from build123d import *

# Parameters (mm, degrees)
SKETCH1_W                = 15.621
SKETCH1_H                = 20.193
SKETCH1_R                = 1.7145
BOSS_EXTRUDE1_DEPTH      = 1.3
SKETCH2_R                = 1.7145
BOSS_EXTRUDE2_DEPTH      = 3.6
BOSS_EXTRUDE2_DRAFT      = 3
SKETCH3_W                = 2
SKETCH3_H                = 2.155291512
SKETCH3_H_2              = 4
SKETCH3_W_2              = 1.5
SKETCH3_H_3              = 2.998822354
BOSS_EXTRUDE3_DEPTH      = 0.3
BOSS_EXTRUDE3_DEPTH_BACK = 0.3


with BuildPart() as part:
    # Sketch1 → Boss-Extrude1 (new body)
    with BuildSketch(Plane(origin=(0, 0, 0), x_dir=(1, 0, 0), z_dir=(0, 1, 0))):
        with Locations((7.8105, 10.0965)):
            Rectangle(SKETCH1_W, SKETCH1_H)
        with Locations((7.8105, 14.4785)):
            Circle(SKETCH1_R, mode=Mode.SUBTRACT)
    extrude(amount=BOSS_EXTRUDE1_DEPTH)


with BuildPart() as boss_extrude2_tool:
    # Sketch2 → Boss-Extrude2 (with draft: the straight prism first)
    with BuildSketch(Plane(origin=(0, 1.3, 0), x_dir=(1, 0, 0), z_dir=(0, 1, 0))):
        with BuildLine():
            Line((15.621, 20.193), (0, 20.193))
            Line((0, 20.193), (0, 17.3995))
            ThreePointArc((0, 17.3995), (2.065458908, 16.543958908), (2.921, 14.4785))
            ThreePointArc((2.921, 14.4785), (2.065458908, 12.413041092), (0, 11.5575))
            Line((0, 11.5575), (0, 0))
            Line((0, 0), (15.621, 0))
            Line((15.621, 0), (15.621, 11.5575))
            ThreePointArc((15.621, 11.5575), (12.7, 14.4785), (15.621, 17.3995))
            Line((15.621, 17.3995), (15.621, 20.193))
        make_face()
        with Locations((7.8105, 14.4785)):
            Circle(SKETCH2_R, mode=Mode.SUBTRACT)
    extrude(amount=BOSS_EXTRUDE2_DEPTH)
    # Boss-Extrude2: the draft: its side faces are tilted about the plane it starts from
    boss_extrude2_sides = [boss_extrude2_tool.faces().sort_by_distance(p)[0] for p in [
        (15.621, 3.1, -18.79625),
        (6.096, 3.1, -14.4785),
        (15.621, 3.1, -5.77875),
        (7.8105, 3.1, 0),
        (0, 3.1, -5.77875),
        (2.921, 3.1, -14.4785),
        (0, 3.1, -18.79625),
        (7.8105, 3.1, -20.193),
        (12.7, 3.1, -14.4785),
    ]]
    draft(boss_extrude2_sides, Plane(origin=(0, 1.3, 0), x_dir=(1, 0, 0), z_dir=(0, 1, 0)), BOSS_EXTRUDE2_DRAFT)


with BuildPart() as part_1:
    add(part.part)

    # Boss-Extrude2: add boss_extrude2_tool
    add(boss_extrude2_tool.part)

    # Sketch3 → Boss-Extrude3 (add, two sides)
    with BuildSketch(Plane(origin=(0, 2.45, 0), x_dir=(1, 0, 0), z_dir=(0, 1, 0))) as boss_extrude3_sk:
        with Locations((2.8105, 1.077645756)):
            Rectangle(SKETCH3_W, SKETCH3_H)
        with Locations((2.8105, -2)):
            Rectangle(SKETCH3_W, SKETCH3_H_2)
        with Locations((12.8105, 1.077645756)):
            Rectangle(SKETCH3_W, SKETCH3_H)
        with Locations((12.8105, -2)):
            Rectangle(SKETCH3_W, SKETCH3_H_2)
        with Locations((7.0605, 1.499411177)):
            Rectangle(SKETCH3_W_2, SKETCH3_H_3)
        Polygon((7.8105, 0), (6.3105, 0), (6.3105, -4), (9.3105, -4), (9.3105, 0), align=None)
        with Locations((8.5605, 1.499411177)):
            Rectangle(SKETCH3_W_2, SKETCH3_H_3)
    extrude(amount=BOSS_EXTRUDE3_DEPTH)
    extrude(boss_extrude3_sk.sketch, amount=-BOSS_EXTRUDE3_DEPTH_BACK)


solid = part_1.part
Can you work these out from the model? Positions are in its coordinate system, mm. A direction names the side the tool comes from. Coordinates: 2 decimals unless noted, no trailing zeros. Order: outer loops, then holes, each group sorted by start corner. A loop starts at its lowest first (then second) coordinate and runs counter-clockwise, first axis right, second up. Notation, with made-up numbers: M -39,1.5 L -11,1.5 A25 ccw -11,16.5 Z; hole C 36,11 d8. An arc over 180 degrees is marked long. Write item = value, one per line.
(1) Suppose I cut it at C-C on y = 0.8. Please give me the cut outline in (x, z) (1 decimal).
Results are:
outline = M 0,-20.2 L 15.6,-20.2 L 15.6,0 L 0,0 Z; hole C 7.8,-14.5 d3.4
(2) I need wall thicknesses on line 1 along X through (y, z) = (2.55, -15.5); line 2 along Z through (x, y) = (14, 2.35); line 3 along Z through (x, y) = (13.25, 2.8). Which ranges of each line are inside material? Lowest first, please. Write a range as [from, to].
Results are:
line_1 = [2.81, 6.35], [9.27, 12.81]
line_2 = [-20.14, -16.97], [-11.98, -0.06]
line_3 = [-20.11, -16.32], [-12.64, -0.08]
(3) If we mould it in two halves opening along Z, with no side actions, what happens to faces 5 (the face through (8.602, 0.641, -12.957)), 6 (the face through (13, 2.75, 2)), 7 (the face through (8, 1, -20.193)), 8 (the face through (12.61, 3.07, -14.41))? For each: pulls with the +Z half, pulls with the -Z half, needs draft (parallel to the pull), parting line crosses it, or undercut.
Results are:
face_5 = undercut
face_6 = needs draft
face_7 = pulls with the -Z half
face_8 = undercut
(4) For faces 1 (the face through (1, 1.3, -15)), 2 (the face through (3, 2.75, 2)), 3 (the face through (15.53, 3.07, -5.7)), 4 (the face through (8, 1, 0)), which set-ups out of +Z, -Z, +X, -X, +Y, -Y let a thin tool reach every point of the face, with its end or its side?
Results are:
face_1 = -X, +Y
face_2 = +Z, +X, -X, +Y
face_3 = +Z, -Z, +X, +Y
face_4 = +Z, +X, -X, -Y
(5) For pin 1 Ø1.4 at (x, y) = (7.5, 0.5) entering from +Z; pin 2 Ø1.5 at (x, z) = (14.5, -15) entering from +Y; pin 3 Ø2 at (x, z) = (7.81, -14.48) entering from +Y; pin 4 Ø1.6 at (x, z) = (12.5, 1) entering from -Y, each with a flat end and sliding along its axis, tell me the tip position at first contact or that it passes through.
Results are:
pin_1 = 0
pin_2 = 1.3
pin_3 = through
pin_4 = 2.15
(6) Suppose I cut it at B-B on x = 11.5. Please give me the cut outline in (y, z), plus the area to 3 significant figures.
Results are:
outline = M 0,-20.19 L 1.3,-20.19 L 4.9,-20 L 4.9,-0.19 L 1.3,0 L 0,0 Z
area = 98.3 mm2
